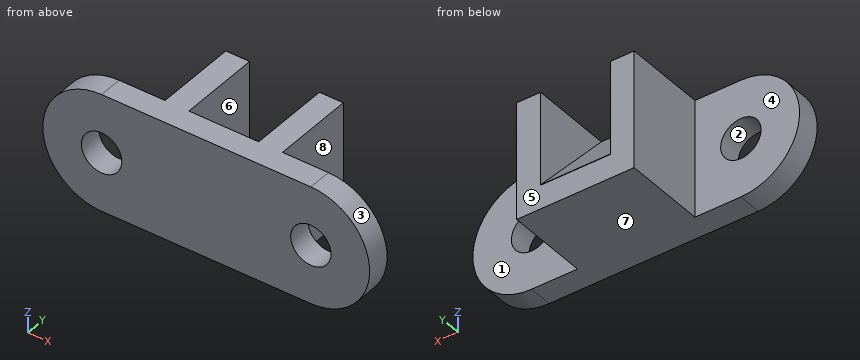
```python
from build123d import *

# Parameters (mm, degrees)
SKETCH2_R           = 11
BOSS_EXTRUDE1_DEPTH = 58
CUT_EXTRUDE1_START  = -45
CUT_EXTRUDE1_DEPTH  = 45
SKETCH4_W           = 38
SKETCH4_H           = 51
CUT_EXTRUDE7_DEPTH  = 45
BOSS_EXTRUDE2_DEPTH = 45


with BuildPart() as part:
    # Sketch2 → Boss-Extrude1 (new body)
    with BuildSketch(Plane(origin=(0, 0, 0), x_dir=(1, 0, 0), z_dir=(0, 1, 0))):
        with BuildLine():
            Line((57, 32), (-57, 32))
            ThreePointArc((-57, 32), (-89, 0), (-57, -32))
            Line((-57, -32), (57, -32))
            ThreePointArc((57, -32), (89, 0), (57, 32))
        make_face()
        with Locations(Location((-57, 0, 0), (0, 0, 90))):
            Circle(SKETCH2_R, mode=Mode.SUBTRACT)
        with Locations(Location((57, 0, 0), (0, 0, 90))):
            Circle(SKETCH2_R, mode=Mode.SUBTRACT)
    extrude(amount=BOSS_EXTRUDE1_DEPTH)

    # Sketch3 → Cut-Extrude1 (cut)
    with BuildSketch(Plane(origin=(0, 58, 0), x_dir=(1, 0, 0), z_dir=(0, 1, 0)).offset(CUT_EXTRUDE1_START)):
        with BuildLine():
            Line((-32, 32), (-32, -32))
            Line((-32, -32), (-57, -32))
            ThreePointArc((-57, -32), (-89, 0), (-57, 32))
            Line((-57, 32), (-32, 32))
        make_face()
        with BuildLine():
            Line((32, 32), (32, -32))
            Line((32, -32), (57, -32))
            ThreePointArc((57, -32), (89, 0), (57, 32))
            Line((57, 32), (32, 32))
        make_face()
    extrude(amount=CUT_EXTRUDE1_DEPTH, mode=Mode.SUBTRACT)

    # Sketch4 → Cut-Extrude7 (cut)
    with BuildSketch(Plane(origin=(0, 58, 0), x_dir=(1, 0, 0), z_dir=(0, 1, 0))):
        with Locations((0, -6.5)):
            Rectangle(SKETCH4_W, SKETCH4_H)
    extrude(amount=-CUT_EXTRUDE7_DEPTH, mode=Mode.SUBTRACT)

    # Sketch6 → Boss-Extrude2 (add)
    with BuildSketch(Plane(origin=(-19, 0, 0), x_dir=(0, 0, -1), z_dir=(1, 0, 0))):
        Polygon((18.765593609, 58), (-32, 13), (18.765593609, 13), align=None)
    extrude(amount=BOSS_EXTRUDE2_DEPTH)


solid = part.part
```
The listing builds one solid part. Answer for the finished solid, in the listing's coordinates (mm). Face numbers are marked on the shaded views. A direction names the side the tool comes from. Coordinates: 2 decimals unless noted, no trailing zeros. Write each loop counter-clockwise with the first axis right and the second up, starting at its lowest first coordinate (ties: lowest second). Pieces come first, ordered by that corner, then holes.
Q1. Find the intervals of material crossed by line 1 along X through (y, z) = (7.25, 0); line 2 along Z through (x, y) = (57, 4); line 3 along Y through (x, z) = (72.5, -6.5), in increasing order.
Returned:
line 1: x = -89 to -68, -46 to 46, 68 to 89
line 2: z = -32 to -11, 11 to 32
line 3: y = 0 to 13
Q2. The mould has two halves that part along X. Classify the marked faces 1, 2 and 3: released by +X, released by -X, zero draft, split by the parting line, or undercut.
Returned:
face 1: zero draft
face 2: undercut
face 3: released by +X
Q3. Section A-A, the plane y = 8 is taken. Write down the section's boundary in (x, z), then the cut area to 3 significant figures.
Returned:
outline: (-57, -32) - (57, -32) arc R32 ccw to (57, 32) - (-57, 32) arc R32 ccw to start; hole circle Ø22 at (-57, 0); hole circle Ø22 at (57, 0)
area: 9,750 mm2
Q4. Section B-B, the plane x = 63.5 is taken. Write down the section's boundary in (y, z).
Returned:
outline: (0, -31.33) - (13, -31.33) - (13, -8.87) - (0, -8.87) - close; (0, 8.87) - (13, 8.87) - (13, 31.33) - (0, 31.33) - close
Q5. Section D-D, the plane y = 18 is taken. Write down the section's boundary in (x, z), then the cut area to 3 significant figures.
Returned:
outline: (-32, -32) - (32, -32) - (32, 32) - (19, 32) - (19, 26.36) - (-19, 26.36) - (-19, 32) - (-32, 32) - close; hole (-19, -19) - (19, -19) - (19, -18.77) - (-19, -18.77) - close
area: 3,870 mm2
Q6. Given P1, Ø10, axis at y = 39.5, z = 5, coming from the +X side; P2, Ø5, axis at y = 27, z = 22.5, coming from the -X side; P3, Ø17, axis at x = 67.5, z = -10, coming from the +Y side, each flat-ended and moving along its own axis, determine where each tip first touches the part or whether it passes through.
Returned:
P1: stops at x = 32
P2: stops at x = -32
P3: stops at y = 13
Q7. Section C-C, the plane z = 5.5 is taken. Write down the section's boundary in (x, y), then the cut area to 3 significant figures.
Returned:
outline: (-88.52, 0) - (-66.53, 0) - (-66.53, 13) - (-88.52, 13) - close; (-47.47, 0) - (47.47, 0) - (47.47, 13) - (32, 13) - (32, 58) - (19, 58) - (19, 36.49) - (-19, 36.49) - (-19, 58) - (-32, 58) - (-32, 13) - (-47.47, 13) - close; (66.53, 0) - (88.52, 0) - (88.52, 13) - (66.53, 13) - close
area: 3,870 mm2
Q8. Which of the six approach directions +Z, -Z, +X, -X, +Y, -Y give full straight-line access (tool end or side, diameter ignored) to the marked faces 4, 5, 6, 7 and 8?
Returned:
face 4: +Z, -Z, -X, +Y
face 5: +Z, -Z, +X, -X, +Y
face 6: +Z, +Y
face 7: -Z, +X, -X, +Y, -Y
face 8: +Z, -Z, +X, +Y
